from build123d import *

# Parameters (mm, degrees)
SKETCH2_W                    = 60
SKETCH2_H                    = 29.1
BASE_FLANGE1_DEPTH           = 4
EDGE_FLANGE1_STRIP_W         = 26
EDGE_FLANGE1_STRIP_H         = 4
EDGE_FLANGE1_STRIP_CUT_DEPTH = 60
EDGE_FLANGE1_DEPTH           = 60
EDGE_FLANGE2_STRIP_W         = 26
EDGE_FLANGE2_STRIP_H         = 4
EDGE_FLANGE2_STRIP_CUT_DEPTH = 60
EDGE_FLANGE2_DEPTH           = 60
F_1_0MM_DOWEL_HOLE1_D        = 5
LPATTERN1_COUNT              = 6
LPATTERN1_PITCH              = 10
LPATTERN1_COUNT_DIR2         = 5
LPATTERN1_PITCH_DIR2         = 10
FILLET1_R                    = 5


# Sheet-metal steps are written as plain solids
with BuildPart() as part:
    # Sketch2 → Base-Flange1 (new body)
    with BuildSketch(Plane(origin=(0, 0, 0), x_dir=(1, 0, 0), z_dir=(0, 1, 0))):
        Rectangle(SKETCH2_W, SKETCH2_H)
    extrude(amount=-BASE_FLANGE1_DEPTH)

    # Edge-Flange1 strip (across the edge) → Edge-Flange1 strip cut (cut)
    with BuildSketch(Plane(origin=(-30, 0, 14.55), x_dir=(0, 0, -1), z_dir=(1, 0, 0))):
        with Locations((-8, -2)):
            Rectangle(EDGE_FLANGE1_STRIP_W, EDGE_FLANGE1_STRIP_H)
    extrude(amount=EDGE_FLANGE1_STRIP_CUT_DEPTH, mode=Mode.SUBTRACT)

    # Edge-Flange1 section (across the edge) → Edge-Flange1 (add)
    with BuildSketch(Plane(origin=(-30, 0, 14.55), x_dir=(0, 0, -1), z_dir=(1, 0, 0))):
        with BuildLine():
            Line((-4, 5), (-4, 62))
            Line((-4, 62), (0, 62))
            Line((0, 62), (0, 5))
            ThreePointArc((0, 5), (1.464466094, 1.464466094), (5, 0))
            Line((5, 0), (5, -4))
            ThreePointArc((5, -4), (-1.363961031, -1.363961031), (-4, 5))
        make_face()
    extrude(amount=EDGE_FLANGE1_DEPTH)

    # Edge-Flange2 strip (across the edge) → Edge-Flange2 strip cut (cut)
    with BuildSketch(Plane(origin=(30, 0, -14.55), x_dir=(0, 0, 1), z_dir=(-1, 0, 0))):
        with Locations((-8, -2)):
            Rectangle(EDGE_FLANGE2_STRIP_W, EDGE_FLANGE2_STRIP_H)
    extrude(amount=EDGE_FLANGE2_STRIP_CUT_DEPTH, mode=Mode.SUBTRACT)

    # Edge-Flange2 section (across the edge) → Edge-Flange2 (add)
    with BuildSketch(Plane(origin=(30, 0, -14.55), x_dir=(0, 0, 1), z_dir=(-1, 0, 0))):
        with BuildLine():
            Line((-4, 5), (-4, 61))
            Line((-4, 61), (0, 61))
            Line((0, 61), (0, 5))
            ThreePointArc((0, 5), (1.464466094, 1.464466094), (5, 0))
            Line((5, 0), (5, -4))
            ThreePointArc((5, -4), (-1.363961031, -1.363961031), (-4, 5))
        make_face()
    extrude(amount=EDGE_FLANGE2_DEPTH)

    # Ø1.0mm Dowel Hole1 (through all)
    with Locations(Plane(origin=(0, 0, -18.55), x_dir=(-1, 0, 0), z_dir=(0, 0, -1))):
        with Locations((-25, 56)):
            f_1_0mm_dowel_hole1 = Hole(F_1_0MM_DOWEL_HOLE1_D / 2)

    # LPattern1: 1.0mm Dowel Hole1 6 × 5
    with Locations(*[(-i * LPATTERN1_PITCH, -j * LPATTERN1_PITCH_DIR2, 0) for i in range(LPATTERN1_COUNT) for j in range(LPATTERN1_COUNT_DIR2) if (i, j) != (0, 0)]):
        add(f_1_0mm_dowel_hole1, mode=Mode.SUBTRACT)

    # Fillet1
    fillet1_edges = [part.edges().sort_by_distance(p)[0] for p in [
        (-30, 62, 16.55),
        (30, 62, 16.55),
        (30, 61, -16.55),
        (-30, 61, -16.55),
    ]]
    fillet(fillet1_edges, radius=FILLET1_R)


solid = part.part
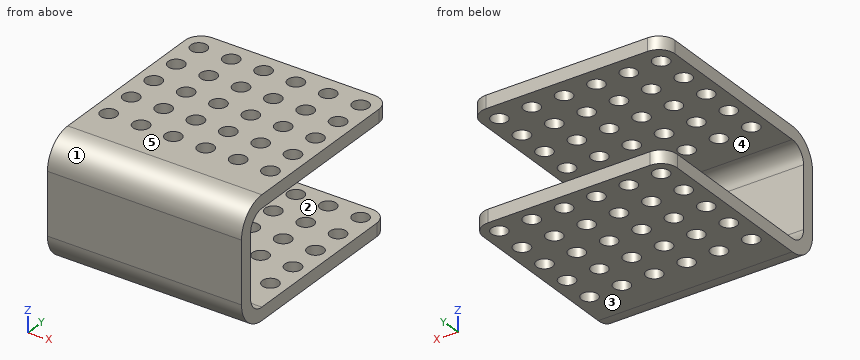
The listing builds one solid part. Answer for the finished solid, in the listing's coordinates (mm). Face numbers are marked on the shaded views. A direction names the side the tool comes from. Round coordinates to 2 decimals unless told otherwise and drop trailing zeros. Order: outer loops, then holes, each group sorted by start corner. A loop starts at its lowest first (then second) coordinate and runs counter-clockwise, first axis right, second up. Notation, with made-up numbers: (-3.75, 1.25) -> (3.25, 1.25) arc R24 cw to (3.25, 18.25) -> close; hole circle Ø4 at (-10, 70). An arc over 180 degrees is marked (long way). One line per item, written item: value.
Item 1: Straight lines are drawn through the part: L1, parallel to Z at x = -6.5, y = 59.5; L2, parallel to Y at x = 25, z = -16.2. For each, find the intervals that lie inside material, in ascending order.
Taken from the geometry:
L1: z = -18.55 to -14.55, 14.55 to 18.55
L2: y = -1.06 to 13.5, 18.5 to 23.5, 28.5 to 33.5, 38.5 to 43.5, 48.5 to 53.5, 58.5 to 61
Item 2: Find section A-A, the plane y = 9.5. Give the vertices of the cut face in (x, z), then the cut area to 3 significant figures.
Taken from the geometry:
outline: (-30, -18.55) -> (30, -18.55) -> (30, -14.55) -> (-30, -14.55) -> close; (-30, 14.55) -> (30, 14.55) -> (30, 18.55) -> (-30, 18.55) -> close
area: 480 mm2
Item 3: For a pull along Z with two mould halves and no side action, classify the marked faces 1, 2 and 3 as released by +Z, released by -Z, zero draft, split by the parting line, or undercut.
Taken from the geometry:
face 1: released by +Z
face 2: undercut
face 3: released by -Z
Item 4: Find section B-B, the plane x = -9. Give the vertices of the cut face in (y, z).
Taken from the geometry:
outline: (-4, -9.55) arc R9 ccw to (5, -18.55) -> (61, -18.55) -> (61, -14.55) -> (5, -14.55) arc R5 cw to (0, -9.55) -> (0, 9.55) arc R5 cw to (5, 14.55) -> (62, 14.55) -> (62, 18.55) -> (5, 18.55) arc R9 ccw to (-4, 9.55) -> close
Item 5: Given P1, Ø21, axis at x = 14, z = 3.5, coming from the +Y side; P2, Ø8, axis at x = 5, y = 46, coming from the -Z side; P3, Ø3, axis at x = 15, y = 26, coming from the -Z side; P4, Ø3, axis at x = 13, z = -13, coming from the -Y side, each flat-ended and moving along its own axis, determine where each tip first touches the part or whether it passes through.
Taken from the geometry:
P1: stops at y = 2.72
P2: stops at z = -18.55
P3: passes through
P4: stops at y = -3.79
Item 6: For the marked faces 4 and 5, determine the directions among +Z, -Z, +X, -X, +Y, -Y from which every point of the face is accessible in a straight line to the end or side of a thin tool.
Taken from the geometry:
face 4: +X, -X, +Y
face 5: +Z, +X, -X, +Y, -Y
Item 7: Find section C-C, the plane x = 15. State how many separate pieces and enclosed holes the cut face has, then the cut area to 3 significant figures.
Taken from the geometry:
separate pieces: 11
enclosed holes: 0
area: 416 mm2
